Autodesk Inventor part; units mm, degrees
ref_plane "XY Plane" through (0, 0, 0) normal (0, 0, 1) x (1, 0, 0)
sketch "Sketch1" plane through (0, 0, 0) normal (0, 1, 0) x (-1, 0, 0)
  circle A0 centre (0, 0) radius 12.612
  line L0 (12.612, 0) -> (-12.612, 0)
  circle A1 centre (0, 0) radius 21.59
  dimension "d29" = 43.18
revolve "Revolution1" add sketch "Sketch1" angle 360 about axis through (-12.612, 0, 0) along (1, 0, 0) contours L0 A0 | A0 L0
sketch "Sketch2" plane through (0, 0, 0) normal (0, 1, 0) x (-1, 0, 0)
  circle A0 centre (0, 0) radius 6.3549
extrude "Extrusion1" cut sketch "Sketch2" along normal mid plane 25.4
hole "Hole1" [suppressed]
hole "Hole2" [suppressed]
sketch "Sketch3" plane through (0, 0, 0) normal (0, 1, 0) x (-1, 0, 0)
  point P0 (0, 0)
sketch "Sketch4" plane through (0, 0, 0) normal (1, 0, 0) x (0, 1, 0)
  line L0 (6.604, 13.4644) -> (-12.0538, 13.4644)
  line L1 (-12.0538, 13.4644) -> (-12.0538, -13.0797)
  line L2 (-12.0538, -13.0797) -> (6.604, -13.0797)
  line L3 (6.604, -13.0797) -> (6.604, 13.4644)
  point P0 (0, 0)
extrude "Extrusion2" cut sketch "Sketch4" along normal mid plane 30.48
sketch "Sketch5" plane through (0, 0, 0) normal (1, 0, 0) x (0, 1, 0)
  circle A0 centre (0, 0) radius 8.7198
extrude "Extrusion3" cut sketch "Sketch5" along normal mid plane 30.48
sketch "Sketch6" plane through (0, 0, 0) normal (0, 1, 0) x (-1, 0, 0)
  circle A0 centre (0, 0) radius 6.3549
  circle A1 centre (0, 0) radius 7.0528
extrude "Extrusion4" add sketch "Sketch6" along normal blind 11.176
sketch "Sketch7" plane through (0, 0, 0) normal (0, 1, 0) x (-1, 0, 0)
  circle A0 centre (0, 0) radius 6.3549
  circle A1 centre (0, 0) radius 7.0528
extrude "Extrusion5" cut sketch "Sketch7" along normal blind 10.16
sketch "Sketch8" plane through (0, 0, 0) normal (0, 1, 0) x (-1, 0, 0)
  point P0 (0, 0)
sketch "Sketch9" plane through (0, 0, 0) normal (0, 1, 0) x (-1, 0, 0)
  circle A0 centre (0, 0) radius 12.319
  line L0 (12.319, 0) -> (-12.319, 0)
  dimension "d30" = 24.638
revolve "Revolution2" cut sketch "Sketch9" angle 360 about axis through (-12.319, 0, 0) along (1, 0, 0)
properties part number "side"
For this review, take the finished solid that the model builds, in its own axes (mm). Round coordinates to 2 decimals unless told otherwise and drop trailing zeros. Loops run counter-clockwise (first coordinate to the right, second up) from the corner with the lowest first, then second, coordinate; pieces in that order, holes last. Notation, with made-up numbers: (-32, 79) - (2, 79) arc R18 cw to (2, 108) - close; hole circle Ø5 at (-29, -17.5). An arc over 180 degrees is marked (long way). One line per item, written item: value. Start each with the question number.
Item 1: Clearance check with flat-ended pins moving along their axes: pin 1 Ø10 at (x, z) = (2, -4) entering from -Y; pin 2 Ø7 at (x, z) = (-0.5, -1.5) entering from -Y. State where each tip first meets the part, or that it passes through.
Item 2: Take a section at B-B (z = 0). Give the boundary of the cut face in (x, y), plus the area to 3 significant figures.
Item 3: The part is to be moulded in two halves that separate along Z. For faces 1 (the flat face through (6, 11.176, 3)), 2 (the cylindrical face through (8.9, 8.72, 0.09)), 3 (the cylindrical face through (1.529, 10.811, 6.885)), say which applies: +Z half, -Z half, draft (parallel to the pull), parting line (faces both ways), or undercut.
Item 4: For L1, parallel to Z at x = 0, y = 10.8; L2, parallel to Z at x = 1.5, y = 10.5; L3, parallel to X at y = 10.7, z = 3.25, list the stretches that pass through material, from the lowest coordinate up.
Item 5: Take a section at D-D (y = 9.05). Give the boundary of the cut face in (x, z).
Item 6: Take a section at A-A (x = 0). Give the boundary of the cut face in (y, z), plus the area to 3 significant figures.
Item 7: Take a section at C-C (y = 7.1). Give the boundary of the cut face in (x, z), plus the area to 3 significant figures.
Answer below:
1. pin 1: stops at y = 7.88
1. pin 2: passes through
2. outline: (-9.11, 8.72) - (-8.7, 8.72) arc R12.32 cw to (-7.05, 10.1) - (-7.05, 10.16) - (-6.97, 10.16) arc R12.32 cw to (-6.35, 10.55) - (-6.35, 11.18) - (-7.05, 11.18) - (-7.05, 10.46) arc R12.61 ccw to start; (6.35, 10.55) arc R12.32 cw to (6.97, 10.16) - (7.05, 10.16) - (7.05, 10.1) arc R12.32 cw to (8.7, 8.72) - (9.11, 8.72) arc R12.61 ccw to (7.05, 10.46) - (7.05, 11.18) - (6.35, 11.18) - close
2. area: 2.59 mm2
3. face 1: draft
3. face 2: undercut
3. face 3: parting line
4. L1: z = -7.05 to -6.35, 6.35 to 7.05
4. L2: z = -6.89 to -6.27, 6.27 to 6.89
4. L3: x = -6.26 to -5.46, 5.46 to 6.26
5. outline: circle Ø17.57 at (0, 0); hole circle Ø16.72 at (0, 0)
6. outline: (6.6, -10.74) arc R12.61 ccw to (10.46, -7.05) - (11.18, -7.05) - (11.18, -6.35) - (10.55, -6.35) arc R12.32 cw to (10.16, -6.97) - (10.16, -7.05) - (10.1, -7.05) arc R12.32 cw to (6.6, -10.4) - close; (6.6, 10.4) arc R12.32 cw to (10.1, 7.05) - (10.16, 7.05) - (10.16, 6.97) arc R12.32 cw to (10.55, 6.35) - (11.18, 6.35) - (11.18, 7.05) - (10.46, 7.05) arc R12.61 ccw to (6.6, 10.74) - close
6. area: 4.18 mm2
7. outline: (-9.11, -5.06) arc R10.42 ccw to (9.11, -5.06) - (8.7, -5.06) arc R10.07 cw to (-8.7, -5.06) - close; (-9.11, 5.06) - (-8.7, 5.06) arc R10.07 cw to (8.7, 5.06) - (9.11, 5.06) arc R10.42 ccw to start
7. area: 15.4 mm2
